For this review, use the dimensioned drawing (mm, ordinates from the lowest corner) and the shaded views. A direction names the side the tool comes from. Coordinates: 2 decimals unless noted, no trailing zeros. Write each loop counter-clockwise with the first axis right and the second up, starting at its lowest first coordinate (ties: lowest second). Pieces come first, ordered by that corner, then holes. Notation, with made-up numbers: (-23.75, 47.25) - (-1.75, 47.25) arc R28 ccw to (-1.75, 68.25) - close; hole circle Ø10 at (-4, 7.5). An arc over 180 degrees is marked (long way). Answer as a JSON object with one key per item and string values.
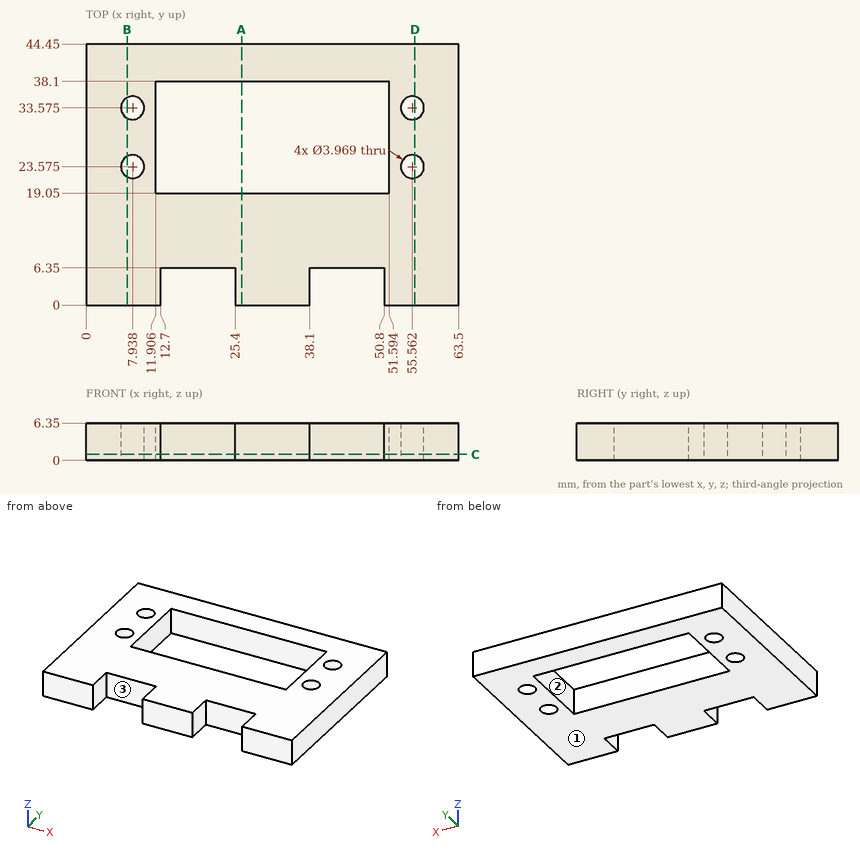
(1) Take a section at C-C, the plane z = 1. Give the number of separate pieces and of enclosed holes in the cut face, and give its area (3 significant figures).
Solved:
{"separate pieces": "1", "enclosed holes": "5", "area": "1,860 mm^2"}
(2) To check wall thickness, follow line 1 (X direction, y = 5, z = 5.75); line 2 (Y direction, x = 34, z = 5); line 3 (Y direction, x = 16.5, z = 0.75). State the ranges of each line that lie inside material, in increasing order. Write a range as from..to.
Solved:
{"line 1": "x = 0..12.7, 25.4..38.1, 50.8..63.5", "line 2": "y = 0..19.05, 38.1..44.45", "line 3": "y = 6.35..19.05, 38.1..44.45"}
(3) For pin 1 (1.9 mm diameter, centred on x = 41.5, z = 2.5, fed in from -Y), flat-tipped, find the tip position at first contact; note if it passes through.
Solved:
{"pin 1": "stops at y = 6.35"}
(4) Take a section at D-D, the plane x = 56. Write out the cut boundary in (y, z).
Solved:
{"outline": "(0, 0) - (21.64, 0) - (21.64, 6.35) - (0, 6.35) - close; (25.51, 0) - (31.64, 0) - (31.64, 6.35) - (25.51, 6.35) - close; (35.51, 0) - (44.45, 0) - (44.45, 6.35) - (35.51, 6.35) - close"}
(5) Tool access review of the marked faces 1, 2 and 3: name each direction out of +Z, -Z, +X, -X, +Y, -Y from which nothing blocks a thin tool from reaching the whole face with its end or side.
Solved:
{"face 1": "-Z, +X, -X, +Y, -Y", "face 2": "+Z, -Z", "face 3": "+Z, -Z, -Y"}
(6) Take a section at B-B, the plane x = 7. Write out the cut boundary in (y, z), and give its area (3 significant figures).
Solved:
{"outline": "(0, 0) - (21.83, 0) - (21.83, 6.35) - (0, 6.35) - close; (25.32, 0) - (31.83, 0) - (31.83, 6.35) - (25.32, 6.35) - close; (35.32, 0) - (44.45, 0) - (44.45, 6.35) - (35.32, 6.35) - close", "area": "238 mm^2"}
(7) Take a section at A-A, the plane x = 26.5. Write out the cut boundary in (y, z).
Solved:
{"outline": "(0, 0) - (19.05, 0) - (19.05, 6.35) - (0, 6.35) - close; (38.1, 0) - (44.45, 0) - (44.45, 6.35) - (38.1, 6.35) - close"}
